Solid Edge part; units mm, degrees
sketch "Sketch1" plane through (0, 0, 0) normal (0, 0, 1) x (1, 0, 0)
  line L0 (3, 0) -> (3, 8.28)
  line L1 (0, 8.28) -> (3, 8.28)
  line L2 (0, 0) -> (0, 8.28)
  line L3 (0, 0) -> (0, -3.72)
  line L4 (0, -3.72) -> (5.67, -3.72)
  line L5 (5.67, -3.72) -> (5.67, -2.67)
  line L6 (5.67, -2.67) -> (3, 0)
revolve "RevolvedProtrusion1" add sketch "Sketch1" angle 360 about axis through (0, 0, 0) along (0, 1, 0)
sketch "Sketch2" plane through (0, 0, 0) normal (1, 0, 0) x (0, 1, 0)
  line L0 (-3.72, 2.7915) -> (-1.52, 2.7915)
  line L1 (0.0917, 0) -> (-1.52, 2.7915)
  line L2 (-3.72, 0) -> (0.0917, 0)
  line L3 (-3.72, 0) -> (-3.72, 2.7915)
revolve "RevolvedCutout1" cut sketch "Sketch2" angle 360 about axis through (0, -4.5, 0) along (0, 1, 0)
sketch "Sketch3" plane through (0, -3.72, 0) normal (0, -1, 0) x (0, 0, 1)
  circle A0 centre (0, 0) radius 2.7915
  line L0 (-2, -1.1547) -> (0, -2.3094)
  line L1 (0, -2.3094) -> (2, -1.1547)
  line L2 (2, -1.1547) -> (2, 1.1547)
  line L3 (2, 1.1547) -> (0, 2.3094)
  line L4 (0, 2.3094) -> (-2, 1.1547)
  line L5 (-2, 1.1547) -> (-2, -1.1547)
extrude "Protrusion1" add sketch "Sketch3" against normal up to next
sketch "Sketch4" plane through (0, 0, 0) normal (0, 0, 1) x (1, 0, 0)
  line L0 (-2.3094, -3.72) -> (0, -3.72)
  line L1 (0, -3.72) -> (0, -3.1012)
  line L2 (0, -3.1012) -> (-2.3094, -3.72)
revolve "RevolvedCutout2" cut sketch "Sketch4" angle 360 about axis through (0, -4.5, 0) along (0, 1, 0)
fillet "Round1" radius 0.25 1 edges at (0, 0, -3)
chamfer "倒斜角_2" distance 0.4 angle 45 1 edges at (0, 8.28, -3)
cosmetic_thread "Thread1"
Read the model definition and answer for the solid it produces. Units are mm, in the model's axes. A direction names the side the tool comes from. Coordinates: 2 decimals unless noted, no trailing zeros. Write each loop counter-clockwise with the first axis right and the second up, starting at its lowest first coordinate (ties: lowest second). Pieces come first, ordered by that corner, then holes. Notation, with made-up numbers: M -9.75,79.25 L 0.25,79.25 A19 ccw 0.25,91.25 Z; hole C 11.5,50.5 d5. An arc over 180 degrees is marked long. Use a Markdown table: item, result.
Q1. The part is cut by section A-A, the plane y = 1.5. Write down the section's boundary in (x, z), then the cut area to 3 significant figures.
Answer block:
| item | result |
|---|---|
| outline | C 0,0 d6 |
| area | 28.3 mm2 |
Q2. Determine the mould class of faces 1 (the face through (-3, 4, 0)), 2 (the face through (-0.043, 0.008, 0.138)), 3 (the face through (0, 8.28, 0)), 4 (the face through (-1.74, -2.41, -0.99)) for opening direction X: released by +X, released by -X, zero draft, split by the parting line, or undercut.
Answer block:
| item | result |
|---|---|
| face 1 | split by the parting line |
| face 2 | undercut |
| face 3 | zero draft |
| face 4 | undercut |
Q3. Straight lines are drawn through the part: L1, parallel to X at y = -1.75, z = 1.5; L2, parallel to Z at x = 2, y = -2.5; L3, parallel to X at y = 2, z = 0. For each, find the intervals that lie inside material, in ascending order. Write a range as [from, to].
Answer block:
| item | result |
|---|---|
| L1 | x = [-4.51, -1.44], [1.44, 4.51] |
| L2 | z = [-5.12, -0.54], [0.54, 5.12] |
| L3 | x = [-3, 3] |
Q4. Which of the six approach directions +Z, -Z, +X, -X, +Y, -Y give full straight-line access (tool end or side, diameter ignored) to faces 5 (the face through (0, -2, -2)), 6 (the face through (3.09, -0.24, 0.97))?
Answer block:
| item | result |
|---|---|
| face 5 | -Y |
| face 6 | +Y |
Q5. Each of these flat-tipped pins is pushed along its axis until it touches: pin 1 Ø1.2 at (x, y) = (0.5, -2.5) entering from +Z; pin 2 Ø1 at (y, z) = (-2, 3.5) entering from +X; pin 3 Ø4 at (y, z) = (7, -3) entering from +X; pin 4 Ø5 at (x, y) = (-2.5, -0.5) entering from -Z. Where does it stop, or does it pass through?
Answer block:
| item | result |
|---|---|
| pin 1 | stops at z = 5.67 |
| pin 2 | stops at x = 4.35 |
| pin 3 | stops at x = 2.83 |
| pin 4 | stops at z = -5.53 |
